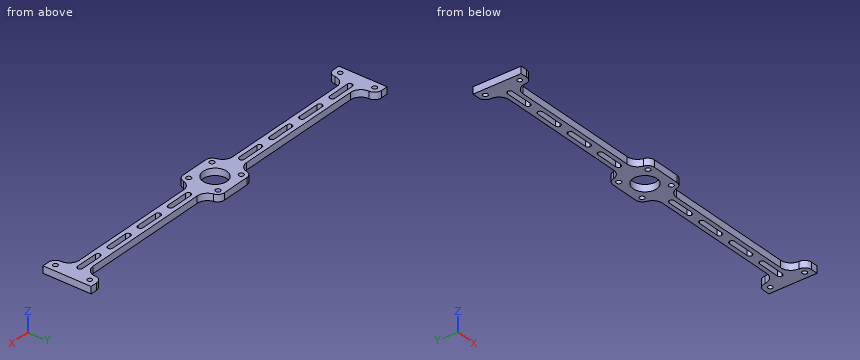
```python
from build123d import *

# Parameters (mm, degrees)
SKETCH4_W            = 139.7
SKETCH4_H            = 12.7
SKETCH4_W_2          = 38.1
BOSS_EXTRUDE2_DEPTH  = 6.35
FILLET4_R            = 9.525
FILLET5_R            = 6.35
SKETCH5_R            = 11
SKETCH5_R_2          = 2.15265
CUT_EXTRUDE1_DEPTH   = 6.35
SKETCH6_R            = 2.2479
CUT_EXTRUDE2_DEPTH   = 6.35
CUT_EXTRUDE3_DEPTH   = 6.35
LPATTERN1_COUNT      = 4
LPATTERN1_PITCH      = 34.925
MIRROR1_COPY_1_DEPTH = 6.35
MIRROR1_COPY_2_DEPTH = 6.35
MIRROR1_COPY_3_DEPTH = 6.35


with BuildPart() as part:
    # Sketch4 → Boss-Extrude2 (new body)
    with BuildSketch(Plane.XY):
        Polygon((-158.75, -22.225), (-158.75, -6.35), (-158.75, 6.35), (-158.75, 22.225), (-171.45, 22.225), (-171.45, -22.225), align=None)
        with Locations((-88.9, 0)):
            Rectangle(SKETCH4_W, SKETCH4_H)
        with Locations((0, 12.7)):
            Rectangle(SKETCH4_W_2, SKETCH4_H)
        Rectangle(SKETCH4_W_2, SKETCH4_H)
        with Locations((0, -12.7)):
            Rectangle(SKETCH4_W_2, SKETCH4_H)
        with Locations((88.9, 0)):
            Rectangle(SKETCH4_W, SKETCH4_H)
        Polygon((158.75, 6.35), (158.75, -6.35), (158.75, -22.225), (171.45, -22.225), (171.45, 22.225), (158.75, 22.225), align=None)
    extrude(amount=BOSS_EXTRUDE2_DEPTH)

    # Fillet4
    fillet4_edges = [part.edges().sort_by_distance(p)[0] for p in [
        (-158.75, 6.35, 3.175),
        (-19.05, 6.35, 3.175),
        (19.05, 6.35, 3.175),
        (158.75, 6.35, 3.175),
        (158.75, -6.35, 3.175),
        (19.05, -6.35, 3.175),
        (-19.05, -6.35, 3.175),
        (-158.75, -6.35, 3.175),
    ]]
    fillet(fillet4_edges, radius=FILLET4_R)

    # Fillet5
    fillet5_edges = [part.edges().sort_by_distance(p)[0] for p in [
        (-158.75, 22.225, 3.175),
        (-158.75, -22.225, 3.175),
        (158.75, -22.225, 3.175),
        (158.75, 22.225, 3.175),
        (19.05, 19.05, 3.175),
        (-19.05, 19.05, 3.175),
        (-19.05, -19.05, 3.175),
        (19.05, -19.05, 3.175),
    ]]
    fillet(fillet5_edges, radius=FILLET5_R - 0.0001)  # a hair under: the kernel refuses the full size

    # Sketch5 → Cut-Extrude1 (cut)
    with BuildSketch(Plane.XY.offset(6.35)):
        Circle(SKETCH5_R)
        with Locations((-165.1, 15.875)):
            Circle(SKETCH5_R_2)
        with Locations((-165.1, -15.875)):
            Circle(SKETCH5_R_2)
        with Locations((165.1, 15.875)):
            Circle(SKETCH5_R_2)
        with Locations((165.1, -15.875)):
            Circle(SKETCH5_R_2)
    extrude(amount=-CUT_EXTRUDE1_DEPTH, mode=Mode.SUBTRACT)

    # Sketch6 → Cut-Extrude2 (cut)
    with BuildSketch(Plane.XY.offset(6.35)):
        with Locations((-13.49375, -13.49375)):
            Circle(SKETCH6_R)
        with Locations((13.49375, -13.49375)):
            Circle(SKETCH6_R)
        with Locations((13.49375, 13.49375)):
            Circle(SKETCH6_R)
        with Locations((-13.49375, 13.49375)):
            Circle(SKETCH6_R)
    extrude(amount=-CUT_EXTRUDE2_DEPTH, mode=Mode.SUBTRACT)

    # Sketch7 → Cut-Extrude3 (cut)
    with BuildSketch(Plane.XY.offset(6.35)):
        with BuildLine():
            Line((-156.369004, 2.38125), (-135.730996005, 2.38125))
            ThreePointArc((-135.730996005, 2.38125), (-134.047377588, 1.683872418), (-133.350000005, 0.000254))
            ThreePointArc((-133.350000005, 0.000254), (-134.047377588, -1.683872418), (-135.730996005, -2.38125))
            Line((-135.730996005, -2.38125), (-156.369004, -2.38125))
            ThreePointArc((-156.369004, -2.38125), (-158.052622418, -1.683872418), (-158.75, 0.000254))
            ThreePointArc((-158.75, 0.000254), (-158.052622418, 1.683872418), (-156.369004, 2.38125))
        make_face()
    cut_extrude3 = extrude(amount=-CUT_EXTRUDE3_DEPTH, mode=Mode.SUBTRACT)

    # LPattern1: Cut-Extrude3 ×4
    with Locations(*[(i * LPATTERN1_PITCH, 0, 0) for i in range(1, LPATTERN1_COUNT)]):
        add(cut_extrude3, mode=Mode.SUBTRACT)

    # Mirror1: Cut-Extrude3 across plane
    add(cut_extrude3.mirror(Plane(origin=(0, 0, 0), x_dir=(0, 0, 1), z_dir=(1, 0, 0))), mode=Mode.SUBTRACT)

    # Mirror1 copy 1 sketch → Mirror1 copy 1 (cut)
    with BuildSketch(Plane(origin=(-34.925, 0, 6.35), x_dir=(-1, 0, 0), z_dir=(0, 0, 1))):
        with BuildLine():
            Line((-156.369004, -2.38125), (-135.730996005, -2.38125))
            ThreePointArc((-135.730996005, -2.38125), (-134.047377588, -1.683872418), (-133.350000005, -0.000254))
            ThreePointArc((-133.350000005, -0.000254), (-134.047377588, 1.683872418), (-135.730996005, 2.38125))
            Line((-135.730996005, 2.38125), (-156.369004, 2.38125))
            ThreePointArc((-156.369004, 2.38125), (-158.052622418, 1.683872418), (-158.75, -0.000254))
            ThreePointArc((-158.75, -0.000254), (-158.052622418, -1.683872418), (-156.369004, -2.38125))
        make_face()
    extrude(amount=-MIRROR1_COPY_1_DEPTH, mode=Mode.SUBTRACT)

    # Mirror1 copy 2 sketch → Mirror1 copy 2 (cut)
    with BuildSketch(Plane(origin=(-69.85, 0, 6.35), x_dir=(-1, 0, 0), z_dir=(0, 0, 1))):
        with BuildLine():
            Line((-156.369004, -2.38125), (-135.730996005, -2.38125))
            ThreePointArc((-135.730996005, -2.38125), (-134.047377588, -1.683872418), (-133.350000005, -0.000254))
            ThreePointArc((-133.350000005, -0.000254), (-134.047377588, 1.683872418), (-135.730996005, 2.38125))
            Line((-135.730996005, 2.38125), (-156.369004, 2.38125))
            ThreePointArc((-156.369004, 2.38125), (-158.052622418, 1.683872418), (-158.75, -0.000254))
            ThreePointArc((-158.75, -0.000254), (-158.052622418, -1.683872418), (-156.369004, -2.38125))
        make_face()
    extrude(amount=-MIRROR1_COPY_2_DEPTH, mode=Mode.SUBTRACT)

    # Mirror1 copy 3 sketch → Mirror1 copy 3 (cut)
    with BuildSketch(Plane(origin=(-104.775, 0, 6.35), x_dir=(-1, 0, 0), z_dir=(0, 0, 1))):
        with BuildLine():
            Line((-156.369004, -2.38125), (-135.730996005, -2.38125))
            ThreePointArc((-135.730996005, -2.38125), (-134.047377588, -1.683872418), (-133.350000005, -0.000254))
            ThreePointArc((-133.350000005, -0.000254), (-134.047377588, 1.683872418), (-135.730996005, 2.38125))
            Line((-135.730996005, 2.38125), (-156.369004, 2.38125))
            ThreePointArc((-156.369004, 2.38125), (-158.052622418, 1.683872418), (-158.75, -0.000254))
            ThreePointArc((-158.75, -0.000254), (-158.052622418, -1.683872418), (-156.369004, -2.38125))
        make_face()
    extrude(amount=-MIRROR1_COPY_3_DEPTH, mode=Mode.SUBTRACT)


solid = part.part
```
Model file for the job. Use its own axes, mm. Coordinates: 2 decimals unless noted, no trailing zeros. Loops run counter-clockwise (first coordinate to the right, second up) from the corner with the lowest first, then second, coordinate; pieces in that order, holes last. Notation, with made-up numbers: (40.25, 74) -> (71.25, 74) arc R18 cw to (71.25, 88) -> close; hole circle Ø6 at (21, -34). An arc over 180 degrees is marked (long way). Answer as a JSON object with one key per item and string values.
Q1. Cut at B-B (x = -75.5). List the corners of the cut face in (y, z), and give its area (3 significant figures).
Report:
{"outline": "(-6.35, 0) -> (-2.38, 0) -> (-2.38, 6.35) -> (-6.35, 6.35) -> close; (2.38, 0) -> (6.35, 0) -> (6.35, 6.35) -> (2.38, 6.35) -> close", "area": "50.4 mm2"}
Q2. Probe probe 1 along Y at (x, z) = (109.5, 1); probe 2 along Y at (x, z) = (-165.1, 2.75) (3 decimals); probe 3 along X at (y, z) = (-9, 4.75). List the from-to ranges inside material, lowest first.
Report:
{"probe 1": "y = -6.35 to -2.38, 2.38 to 6.35", "probe 2": "y = -22.225 to -18.028, -13.722 to 13.722, 18.028 to 22.225", "probe 3": "x = -171.45 to -155.82, -21.98 to -6.32, 6.32 to 21.98, 155.82 to 171.45"}
Q3. Cut at A-A (x = 0). List the corners of the cut face in (y, z).
Report:
{"outline": "(-19.05, 0) -> (-11, 0) -> (-11, 6.35) -> (-19.05, 6.35) -> close; (11, 0) -> (19.05, 0) -> (19.05, 6.35) -> (11, 6.35) -> close"}
Q4. Cut at C-C (x = 59.5). List the corners of the cut face in (y, z).
Report:
{"outline": "(-6.35, 0) -> (6.35, 0) -> (6.35, 6.35) -> (-6.35, 6.35) -> close"}
Q5. Flat gauge pins, fed straight in: P1, Ø1.9, axis at x = 43.5, z = 2.5, coming from the +Y side; P2, Ø1.9, axis at x = -147, z = 1.5, coming from the -Y side; P3, Ø7, axis at x = -165.1, y = 15.875, coming from the -Z side. Where does each tip first touch, or does it go through?
Report:
{"P1": "stops at y = 6.35", "P2": "stops at y = -6.35", "P3": "stops at z = 0"}
Q6. Cut at D-D (z = 3). State how many separate pieces and enclosed holes the cut face has, and give its area (3 significant figures).
Report:
{"separate pieces": "1", "enclosed holes": "17", "area": "4,790 mm2"}
